Input: part model. Units: mm. Frame: model coordinates. Face numbers are marked on the shaded views. Coordinates: 2 decimals unless noted, no trailing zeros. Order: outer loops, then holes, each group sorted by start corner. A loop starts at its lowest first (then second) coordinate and runs counter-clockwise, first axis right, second up. Notation, with made-up numbers: (48, 54) - (107, 54) arc R12 ccw to (107, 58) - close; hole circle Ø3 at (87, 21.25). An arc over 180 degrees is marked (long way). Use a Markdown table: item, result. Add a question column.
Autodesk Inventor part; units mm, degrees
ref_plane "YZ Plane" through (0, 0, 0) normal (1, 0, 0) x (0, 1, 0)
ref_plane "XZ Plane" through (0, 0, 0) normal (0, 1, 0) x (-1, 0, 0)
ref_plane "XY Plane" through (0, 0, 0) normal (0, 0, 1) x (1, 0, 0)
sketch "Sketch1" plane through (0, 0, 0) normal (0, 1, 0) x (-1, 0, 0)
  line L0 (0, 0) -> (14, 0)
  line L1 (14, 0) -> (14, -2)
  line L2 (14, -2) -> (0, -2)
  line L3 (0, -2) -> (0, 0)
  line L4 (14, -1) -> (13, -1)
  line L5 (7, -2) -> (7, -1)
  circle A0 centre (13, -1) radius 0.5
  circle A1 centre (1, -1) radius 0.5
  dimension "d0" = 14
  dimension "d1" = 2
  dimension "d2" = 1
  dimension "d3" = 1
extrude "Extrusion1" add sketch "Sketch1" along normal blind 2
properties part number "link_v3"
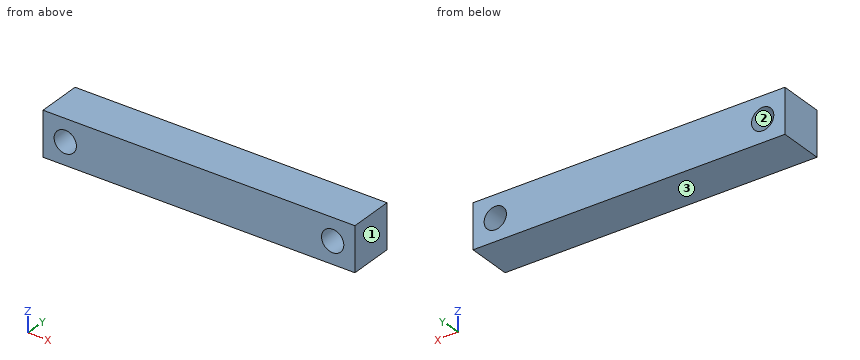
1) Cut plane B-B (x = -1). Return the cut outline in (y, z), and give its area (3 significant figures).
2) Cut plane C-C (y = 1.2). Return the cut outline in (x, z), and give its area (3 significant figures).
3) Material intervals for L1, parallel to X at y = 0.75, z = -1.05; L2, parallel to Z at x = -1, y = 1.2; L3, parallel to X at y = 0.45, z = -0.7, sorted ascending.
4) Cut plane A-A (z = -1). Return the cut outline in (x, y), and give its area (3 significant figures).
5) Pull-direction query (Z, two-part tool) for the marked faces 1, 2 and 3; classes: pulls with the +Z half, pulls with the -Z half, needs draft (parallel to the pull), parting line crosses it, or undercut.
Computed:
| question | item | result |
|---|---|---|
| 1 | outline | (0, -2) - (2, -2) - (2, -1.5) - (0, -1.5) - close; (0, -0.5) - (2, -0.5) - (2, 0) - (0, 0) - close |
| 1 | area | 2.00 mm2 |
| 2 | outline | (-14, -2) - (0, -2) - (0, 0) - (-14, 0) - close; hole circle Ø1 at (-13, -1); hole circle Ø1 at (-1, -1) |
| 2 | area | 26.4 mm2 |
| 3 | L1 | x = -14 to -13.5, -12.5 to -1.5, -0.5 to 0 |
| 3 | L2 | z = -2 to -1.5, -0.5 to 0 |
| 3 | L3 | x = -14 to -13.4, -12.6 to -1.4, -0.6 to 0 |
| 4 | outline | (-14, 0) - (-13.5, 0) - (-13.5, 2) - (-14, 2) - close; (-12.5, 0) - (-1.5, 0) - (-1.5, 2) - (-12.5, 2) - close; (-0.5, 0) - (0, 0) - (0, 2) - (-0.5, 2) - close |
| 4 | area | 24.0 mm2 |
| 5 | face 1 | needs draft |
| 5 | face 2 | undercut |
| 5 | face 3 | pulls with the -Z half |
